Read the model definition and answer for the solid it produces. Units are mm, in the model's axes. A direction names the side the tool comes from. Coordinates: 2 decimals unless noted, no trailing zeros. Loops run counter-clockwise (first coordinate to the right, second up) from the corner with the lowest first, then second, coordinate; pieces in that order, holes last.
Autodesk Inventor part; units mm, degrees
ref_plane "YZ Plane" through (0, 0, 0) normal (1, 0, 0) x (0, 1, 0)
ref_plane "XZ Plane" through (0, 0, 0) normal (0, 1, 0) x (-1, 0, 0)
ref_plane "XY Plane" through (0, 0, 0) normal (0, 0, 1) x (1, 0, 0)
sketch "Sketch1" plane through (0, 0, 0) normal (0, 0, 1) x (1, 0, 0)
  circle A0 centre (0, 0) radius 12.7
  dimension "d0" = 25.4
extrude "Extrusion1" add sketch "Sketch1" along normal blind 5
hole "Hole1" at (0, 0, 5) direction (0, 0, -1) diameter 2.4 depth 2
hole "Hole2" at (0, 0, 3) direction (0, 0, -1) diameter 2 end through all
sketch "Sketch2" plane through (0, 0, 5) normal (0, 0, 1) x (1, 0, 0)
  circle A0 centre (0, 0) radius 12.7
  circle A1 centre (0, 0) radius 7.5
  dimension "d21" = 15
extrude "Extrusion2" add sketch "Sketch2" along normal blind 15
properties part number "Screw_Asm_Jig_Lower"
Item 1: Which of the six approach directions +Z, -Z, +X, -X, +Y, -Y give full straight-line access (tool end or side, diameter ignored) to faces 4 (the face through (1, 0, 1)), 5 (the face through (-7.493, -0.33, 12.395))?
Numbers:
face 4: +Z, -Z
face 5: +Z
Item 2: A cutting plane is placed at D-D on z = 13. Determine the outline of the cut face in (x, y).
Numbers:
outline: circle Ø25.4 at (0, 0); hole circle Ø15 at (0, 0)
Item 3: Determine the mould class of faces 1 (the face through (-2.75, 12.4, 9.86)), 2 (the face through (0, -2, 5)), 3 (the face through (3, 0, 0)) for opening direction X: released by +X, released by -X, zero draft, split by the parting line, or undercut.
Numbers:
face 1: split by the parting line
face 2: undercut
face 3: zero draft
Item 4: A cutting plane is placed at A-A on y = 0. Determine the outline of the cut face in (x, z), then the cut area to 3 significant figures.
Numbers:
outline: (-12.7, 0) - (-1, 0) - (-1, 3) - (-1.2, 3) - (-1.2, 5) - (-7.5, 5) - (-7.5, 20) - (-12.7, 20) - close; (1, 0) - (12.7, 0) - (12.7, 20) - (7.5, 20) - (7.5, 5) - (1.2, 5) - (1.2, 3) - (1, 3) - close
area: 272 mm2
Item 5: Given pin 1 (5 mm diameter, centred on y = 4, z = 8.5, fed in from +X); pin 2 (2.5 mm diameter, centred on x = 0, y = 0.5, fed in from +Z); pin 3 (3 mm diameter, centred on x = 7.5, z = 5, fed in from -Y), each flat-ended and moving along its own axis, determine where each tip first touches the part or whether it passes through.
Numbers:
pin 1: stops at x = 12.61
pin 2: stops at z = 5
pin 3: stops at y = -11.19
Item 6: A cutting plane is placed at C-C on y = 4. Determine the outline of the cut face in (x, z).
Numbers:
outline: (-12.05, 0) - (12.05, 0) - (12.05, 20) - (6.34, 20) - (6.34, 5) - (-6.34, 5) - (-6.34, 20) - (-12.05, 20) - close
Item 7: Find the intervals of material crossed by line 1 along Y through (x, z) = (0, 3.9); line 2 along Y through (x, z) = (0, 14.75); line 3 along Z through (x, y) = (2, 5), in increasing order.
Numbers:
line 1: y = -12.7 to -1.2, 1.2 to 12.7
line 2: y = -12.7 to -7.5, 7.5 to 12.7
line 3: z = 0 to 5
